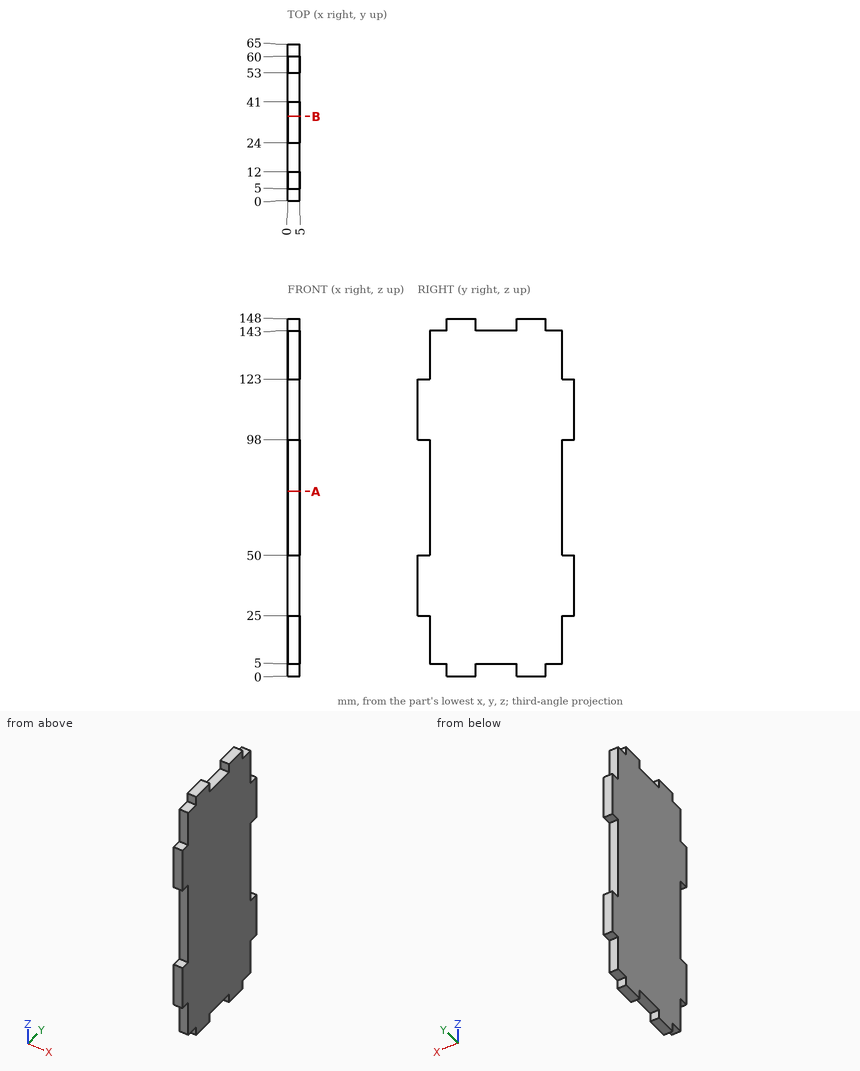
Could you check a few things on this drawing? It's one solid part, dimensions in mm from its lowest x, y, z. Give positions to 0.01 mm unless a question says otherwise; leave off trailing zeros. Write each loop counter-clockwise with the first axis right and the second up, starting at its lowest first coordinate (ties: lowest second). Pieces come first, ordered by that corner, then holes. Notation, with made-up numbers: M 52,-20.5 L 80,-20.5 A13 ccw 80,-11.5 Z; hole C 50,53.5 d4. An arc over 180 degrees is marked long. Put each result on its own line as item: value. Start each with the question number.
Item 1: Will these pins go through, and if not, where does the flat tip stop? pin 1 (1.5 mm diameter, centred on x = 1.5, y = 1.5, fed in from -Z); pin 2 (2.5 mm diameter, centred on x = 2, z = 15.5, fed in from -Y); pin 3 (2.5 mm diameter, centred on x = 2, y = 1.5, fed in from +Z).
Item 2: I need wall thicknesses on L1, parallel to Z at x = 3.7, y = 3.5; L2, parallel to Z at x = 1.85, y = 54; L3, parallel to Y at x = 0.4, z = 130.5. Which ranges of each line are inside material? Lowest first, please. Write a range as from..to.
Item 3: If we section it at A-A, the plane z = 76.5: Write out the boundary of the cut face in (x, y).
Item 4: If we section it at B-B, the plane y = 35: Write out the boundary of the cut face in (x, z).
Values:
1. pin 1: z = 25
1. pin 2: y = 5
1. pin 3: z = 123
2. L1: 25..50, 98..123
2. L2: 5..143
2. L3: 5..60
3. outline: M 0,5 L 5,5 L 5,60 L 0,60 Z
4. outline: M 0,5 L 5,5 L 5,143 L 0,143 Z
